Read the model definition and answer for the solid it produces. Units are mm, in the model's axes. A direction names the side the tool comes from. Coordinates: 2 decimals unless noted, no trailing zeros. Order: outer loops, then holes, each group sorted by start corner. A loop starts at its lowest first (then second) coordinate and runs counter-clockwise, first axis right, second up. Notation, with made-up numbers: (-36.75, 5.25) -> (7.25, 5.25) arc R28 cw to (7.25, 24.25) -> close; hole circle Ø5 at (30.5, 35). An arc over 180 degrees is marked (long way). Answer in a Markdown table with one row per item.
Autodesk Inventor part; units mm, degrees
ref_plane "YZ Plane" through (0, 0, 0) normal (1, 0, 0) x (0, 1, 0)
ref_plane "XZ Plane" through (0, 0, 0) normal (0, 1, 0) x (-1, 0, 0)
ref_plane "XY Plane" through (0, 0, 0) normal (0, 0, 1) x (1, 0, 0)
sketch "Sketch1" plane through (0, 0, 0) normal (0, 0, 1) x (1, 0, 0)
  line L0 (0, 0) -> (0, 1.5875)
  line L1 (0, 1.5875) -> (23.8125, 1.5875)
  line L2 (23.8125, 1.5875) -> (23.8125, 24.2075)
  line L3 (23.8125, 24.2075) -> (25.4, 24.2075)
  line L4 (25.4, 24.2075) -> (25.4, 0)
  line L5 (25.4, 0) -> (0, 0)
  dimension "d0" = 1.5875
  dimension "d3" = 90
  dimension "d9" = 25.4
  dimension "d10" = 22.62
extrude "Extrusion1" add sketch "Sketch1" along normal blind 25.4
sketch "Sketch2" plane through (25.4, 0, 0) normal (1, 0, 0) x (0, 0, -1)
  circle A0 centre (-12.7, 16.7075) radius 7.5
  line L0 (0, 24.2075) -> (-25.4, 24.2075)
  circle A1 centre (-12.7, 16.7075) radius 5
  line L1 (-12.7, 16.7075) -> (-9.4861, 20.5377)
  line L2 (-12.7, 16.7075) -> (-7.776, 15.8393)
  line L3 (-12.7, 16.7075) -> (-10.9899, 12.009)
  line L4 (-12.7, 16.7075) -> (-17.624, 17.5757)
  line L5 (-25.4, 0) -> (-25.4, 24.2075)
  point P0 (0, 0)
  dimension "d6" = 12.7
  dimension "d7" = 7.5
  dimension "d8" = 15
  dimension "d11" = 10
  dimension "d12" = 40
  dimension "d13" = 60
  dimension "d14" = 60
  dimension "d15" = 120
hole "Hole1" at (25.4, 17.5757, 17.624) at (25.4, 20.5377, 9.4861) at (25.4, 15.8393, 7.776) at (25.4, 12.009, 10.9899) direction (-1, 0, 0) diameter 1.5 end through all
sketch "Sketch3" plane through (25.4, 0, 0) normal (1, 0, 0) x (0, 0, -1)
  circle A0 centre (-12.7, 16.7075) radius 7.5
  line L0 (0, 24.2075) -> (-25.4, 24.2075)
  line L1 (0, 24.2075) -> (0, 0)
  dimension "d23" = 15
  dimension "d24" = 7.5
  dimension "d25" = 12.7
hole "Hole2" at (25.4, 16.7075, 12.7) direction (-1, 0, 0) diameter 6 end through all
properties part number "MotorMount" material "Aluminum 6061"
Q1. Given pin 1 (12 mm diameter, centred on y = 20.5, z = 7, fed in from -X), flat-ended and moving along its own axis, determine where the tip first touches the part or whether it passes through.
Outcome:
| item | result |
|---|---|
| pin 1 | x = 23.81 |
Q2. The part is cut by section B-B (z = 23.75). Write down the section's boundary in (x, y).
Outcome:
| item | result |
|---|---|
| outline | (0, 0) -> (25.4, 0) -> (25.4, 24.21) -> (23.81, 24.21) -> (23.81, 1.59) -> (0, 1.59) -> close |
Q3. The part is cut by section C-C (x = 19.25). Write down the section's boundary in (y, z).
Outcome:
| item | result |
|---|---|
| outline | (0, 0) -> (1.59, 0) -> (1.59, 25.4) -> (0, 25.4) -> close |
Q4. Consider line 1 (Y direction, x = 10.5, z = 17.5); line 2 (X direction, y = 7.25, z = 11.5). Determine where each line is inside the solid, lowest interval first.
Outcome:
| item | result |
|---|---|
| line 1 | 0 to 1.59 |
| line 2 | 23.81 to 25.4 |
Q5. The part is cut by section D-D (y = 3.75). Write down the section's boundary in (x, z), then the cut area to 3 significant figures.
Outcome:
| item | result |
|---|---|
| outline | (23.81, 0) -> (25.4, 0) -> (25.4, 25.4) -> (23.81, 25.4) -> close |
| area | 40.3 mm² |
Q6. For a pull along Y with two mould halves and no side action, classify faces 3 (the face through (0, 1, 13)), 4 (the face through (24.595, 21.203, 9.14)), 5 (the face through (13, 0, 13)) as pulls with the +Y half, pulls with the -Y half, needs draft (parallel to the pull), parting line crosses it, or undercut.
Outcome:
| item | result |
|---|---|
| face 3 | needs draft |
| face 4 | undercut |
| face 5 | pulls with the -Y half |
Q7. The part is cut by section A-A (z = 12.7). Write down the section's boundary in (x, y).
Outcome:
| item | result |
|---|---|
| outline | (0, 0) -> (25.4, 0) -> (25.4, 13.71) -> (23.81, 13.71) -> (23.81, 1.59) -> (0, 1.59) -> close; (23.81, 19.71) -> (25.4, 19.71) -> (25.4, 24.21) -> (23.81, 24.21) -> close |
Q8. For faces 1 (the face through (18, 1, 25.4)), 2 (the face through (12, 1.588, 13)), determine the directions among +Z, -Z, +X, -X, +Y, -Y from which every point of the face is accessible in a straight line to the end or side of a thin tool.
Outcome:
| item | result |
|---|---|
| face 1 | +Z, +X, -X, +Y, -Y |
| face 2 | +Z, -Z, -X, +Y |
